Read the model definition and answer for the solid it produces. Units are mm, in the model's axes. Face numbers are marked on the shaded views. A direction names the side the tool comes from. Coordinates: 2 decimals unless noted, no trailing zeros. Order: outer loops, then holes, each group sorted by start corner. A loop starts at its lowest first (then second) coordinate and runs counter-clockwise, first axis right, second up. Notation, with made-up numbers: M 38,15 L 76,15 A9 ccw 76,27 Z; hole C 61.25,-18.75 d4. An arc over 180 degrees is marked long. Write each question's results on one line, items separated by ' | '.
```python
from build123d import *

# Parameters (mm, degrees)
F1_DEPTH = 12.7
F2_W     = 67.376848
F2_H     = 14.811288
F3_DEPTH = 25.4
F4_W     = 67.376848
F4_H     = 45.885952
F5_DEPTH = 5.08
F7_D     = 22.86


with BuildPart() as f1:
    # F0 (on Top) → F1 (new body)
    with BuildSketch(Plane.XY):
        with BuildLine():
            Line((-33.688422, 65.489128), (-33.688422, -55.905353))
            Line((-33.688422, -55.905353), (33.688426, -55.905353))
            Line((33.688426, -55.905353), (33.688426, 66.069968))
            Line((33.688426, 66.069968), (25.84715, 66.069968))
            ThreePointArc((25.84715, 66.069968), (0.308083, 38.360301), (-25.847152, 65.489128))
            Line((-25.847152, 65.489128), (-33.688422, 65.489128))
        make_face()
    extrude(amount=F1_DEPTH)

    # F2 (on face) → F3 (join)
    with BuildSketch(Plane.XY.offset(12.7)):
        with Locations((2e-06, -2.613757)):
            Rectangle(F2_W, F2_H)
    extrude(amount=F3_DEPTH)

    # F4 (on face) → F5 (join)
    with BuildSketch(Plane.XY.offset(12.7)):
        with Locations((2e-06, -32.962377)):
            Rectangle(F4_W, F4_H)
    extrude(amount=F5_DEPTH)

    # F7 (through all)
    with Locations(Plane.XY.offset(17.78)):
        with Locations((0, -29.339861)):
            Hole(F7_D / 2)


solid = f1.part
```
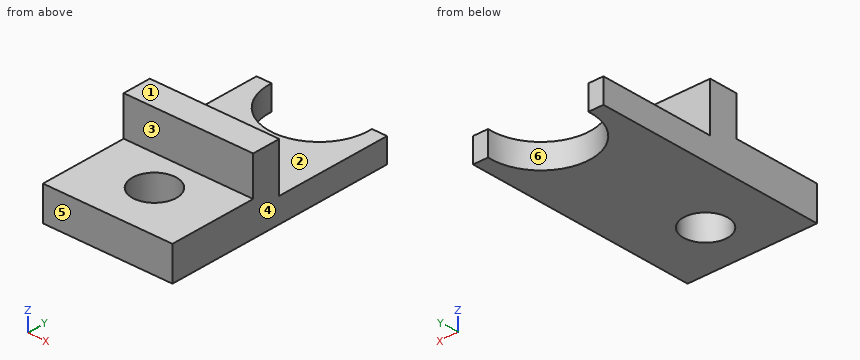
(1) Straight lines are drawn through the part: line 1 (Y direction, x = 0, z = 5); line 2 (Y direction, x = -19, z = 36.5); line 3 (Z direction, x = 25.5, y = 31). For each, find the intervals that lie inside material, in ascending order.
Conclusion:
line 1: -55.91 to -40.77, -17.91 to 38.36 | line 2: -10.02 to 4.79 | line 3: 0 to 12.7
(2) The part is cut by section B-B, the plane y = -20. Write down the section's boundary in (x, z).
Conclusion:
outline: M -33.69,0 L -6.59,0 L -6.59,17.78 L -33.69,17.78 Z; M 6.59,0 L 33.69,0 L 33.69,17.78 L 6.59,17.78 Z
(3) The mould has two halves that part along X. Classify the marked faces 4, 5 and 6: pulls with the +X half, pulls with the -X half, needs draft (parallel to the pull), parting line crosses it, or undercut.
Conclusion:
face 4: pulls with the +X half | face 5: needs draft | face 6: undercut
(4) The part is cut by section A-A, the plane x = 0. Write down the section's boundary in (y, z).
Conclusion:
outline: M -55.91,0 L -40.77,0 L -40.77,17.78 L -55.91,17.78 Z; M -17.91,0 L 38.36,0 L 38.36,12.7 L 4.79,12.7 L 4.79,38.1 L -10.02,38.1 L -10.02,17.78 L -17.91,17.78 Z
(5) The part is cut by section C-C, the plane x = 23. Write down the section's boundary in (y, z), then the cut area to 3 significant figures.
Conclusion:
outline: M -55.91,0 L 52.32,0 L 52.32,12.7 L 4.79,12.7 L 4.79,38.1 L -10.02,38.1 L -10.02,17.78 L -55.91,17.78 Z | area: 1,980 mm²
(6) Given pin 1 (6.5 mm diameter, centred on x = -29, z = 5.5, fed in from +Y); pin 2 (6 mm diameter, centred on x = 2, z = 28, fed in from -Y); pin 3 (8 mm diameter, centred on x = 24.5, z = 17, fed in from +Y), each flat-ended and moving along its own axis, determine where each tip first touches the part or whether it passes through.
Conclusion:
pin 1: y = 65.49 | pin 2: y = -10.02 | pin 3: y = 4.79
(7) The part is cut by section D-D, the plane z = 25. Write down the section's boundary in (x, y), then the cut area to 3 significant figures.
Conclusion:
outline: M -33.69,-10.02 L 33.69,-10.02 L 33.69,4.79 L -33.69,4.79 Z | area: 998 mm²
(8) For the marked faces 1, 2 and 3, determine the directions among +Z, -Z, +X, -X, +Y, -Y from which every point of the face is accessible in a straight line to the end or side of a thin tool.
Conclusion:
face 1: +Z, +X, -X, +Y, -Y | face 2: +Z, +X, -X, +Y | face 3: +Z, +X, -X, -Y
